```python
from build123d import *

# Parameters (mm, degrees)
F0_W     = 8.3
F0_H     = 5
F1_DEPTH = 22.6
F2_W     = 7.9
F2_H     = 8.322741
F2_H_2   = 3.610624
F2_H_3   = 3.642021
F2_H_4   = 3.108276
F2_H_5   = 2.429072
F3_DEPTH = 25
F4_W     = 4.4
F4_H     = 8.322741
F4_H_2   = 3.610624
F4_H_3   = 3.642021
F4_H_4   = 3.108276
F4_H_5   = 2.429072
F5_DEPTH = 25


with BuildPart() as f1:
    # F0 (on Top) → F1 (new body)
    with BuildSketch(Plane.XY):
        with Locations((4.15, -2.5)):
            Rectangle(F0_W, F0_H)
    extrude(amount=F1_DEPTH)

    # F2 (on face) → F3 (cut)
    with BuildSketch(Plane(origin=(0, 0, 0), x_dir=(-1, 0, 0), z_dir=(0, 1, 0))):
        with Locations((-4.15, 18.238629)):
            Rectangle(F2_W, F2_H)
        with Locations((-4.15, 11.86379)):
            Rectangle(F2_W, F2_H_2)
        with Locations((-4.15, 7.9235)):
            Rectangle(F2_W, F2_H_3)
        with Locations((-4.15, 4.234384)):
            Rectangle(F2_W, F2_H_4)
        with Locations((-4.15, 1.214536)):
            Rectangle(F2_W, F2_H_5)
    extrude(amount=-F3_DEPTH, mode=Mode.SUBTRACT)

    # F4 (on Right) → F5 (cut)
    with BuildSketch(Plane.YZ):
        with Locations((-2.5, 18.238629)):
            Rectangle(F4_W, F4_H)
        with Locations((-2.5, 11.86379)):
            Rectangle(F4_W, F4_H_2)
        with Locations((-2.5, 7.9235)):
            Rectangle(F4_W, F4_H_3)
        with Locations((-2.5, 4.234384)):
            Rectangle(F4_W, F4_H_4)
        with Locations((-2.5, 1.214536)):
            Rectangle(F4_W, F4_H_5)
    extrude(amount=F5_DEPTH, mode=Mode.SUBTRACT)


solid = f1.part
```
The model under review builds one solid part; all positions refer to its coordinate system, in mm. Round coordinates to 2 decimals unless told otherwise and drop trailing zeros. Loops run counter-clockwise (first coordinate to the right, second up) from the corner with the lowest first, then second, coordinate; pieces in that order, holes last. Notation, with made-up numbers: M -36.75,87.25 L 22.25,87.25 A23 cw 22.25,105.25 Z; hole C 7.25,36.5 d3. An arc over 180 degrees is marked long. Answer as a JSON object with one key per item and string values.
(1) Take a section at A-A on y = -3.45. Give the boundary of the cut face in (x, z), and give its area (3 significant figures).
Resolved:
{"outline": "M 0,2.43 L 8.3,2.43 L 8.3,2.68 L 0,2.68 Z; M 0,5.79 L 8.3,5.79 L 8.3,6.1 L 0,6.1 Z; M 0,9.74 L 8.3,9.74 L 8.3,10.06 L 0,10.06 Z; M 0,13.67 L 8.3,13.67 L 8.3,14.08 L 0,14.08 Z; M 0,22.4 L 8.3,22.4 L 8.3,22.6 L 0,22.6 Z", "area": "12.3 mm²"}
(2) Take a section at C-C on x = 1.25. Give the boundary of the cut face in (y, z).
Resolved:
{"outline": "M -5,2.43 L 0,2.43 L 0,2.68 L -5,2.68 Z; M -5,5.79 L 0,5.79 L 0,6.1 L -5,6.1 Z; M -5,9.74 L 0,9.74 L 0,10.06 L -5,10.06 Z; M -5,13.67 L 0,13.67 L 0,14.08 L -5,14.08 Z; M -5,22.4 L 0,22.4 L 0,22.6 L -5,22.6 Z"}
(3) To check wall thickness, follow line 1 along Z through (x, y) = (5.5, -2.9). State the ranges of the line that lie inside material, in increasing order.
Resolved:
{"line 1": "2.43 to 2.68, 5.79 to 6.1, 9.74 to 10.06, 13.67 to 14.08, 22.4 to 22.6"}
(4) Take a section at B-B on z = 14.75. Give the boundary of the cut face in (x, y).
Resolved:
{"outline": "M 0,-5 L 0.2,-5 L 0.2,-4.7 L 0,-4.7 Z; M 0,-0.3 L 0.2,-0.3 L 0.2,0 L 0,0 Z; M 8.1,-5 L 8.3,-5 L 8.3,-4.7 L 8.1,-4.7 Z; M 8.1,-0.3 L 8.3,-0.3 L 8.3,0 L 8.1,0 Z"}
